CAD build for the part. Positions are in the model's coordinates, mm. A direction names the side the tool comes from. Give positions to 0.01 mm unless a question says otherwise; leave off trailing zeros. Write each loop counter-clockwise with the first axis right and the second up, starting at its lowest first coordinate (ties: lowest second). Pieces come first, ordered by that corner, then holes. Notation, with made-up numbers: (30.5, 18.5) - (77.5, 18.5) arc R36 cw to (77.5, 56.5) - close; hole circle Ø5 at (43, 64.5). An arc over 180 degrees is marked (long way). Put each result on its own line as item: value. Start each with the question number.
1. Wall check: line 1 (Y direction, x = 0, z = 0.6); line 2 (X direction, y = 12.5, z = 1.7); line 3 (Y direction, x = -21.5, z = 2.8). Give the ranges that are in metal, low to high.
2. Drop flat-ended pins along their axis: pin 1 (1 mm diameter, centred on y = 1.5, z = 0.5, fed in from -X); pin 2 (6.5 mm diameter, centred on x = -20.62, y = 11.91, fed in from -Z); pin 3 (1 mm diameter, centred on x = -0.5, z = 2, fed in from +Y); pin 4 (1 mm diameter, centred on x = -1.5, z = 1.5, fed in from -Y). Give the stop position or say it passes through.
3. Tool access for faces 4 (the flat face through (5.474, 3.219, 1.565)), 5 (the flat face through (0, 7, 0)): list every direction of +Z, -Z, +X, -X, +Y, -Y with a clear straight run to the whole face (end or side of a thin tool).
4. Mould opens along X. For faces 1 (the cylindrical face through (-30.133, 1.326, 1.565)), 2 (the flat face through (0, 7, 3.175)), 3 (the flat face through (5.525, -3.131, 1.565)) say: +X half, -X half, draft (parallel to the pull), parting line (faces both ways), or undercut.
5. Cut at D-D on y = 12.5. List the corners of the cut face in (x, z) (3 decimals).
6. Cut at B-B on y = 4.5. List the corners of the cut face in (x, z) (3 decimals).
7. Cut at A-A on x = 0. Give the number of separate pieces and of enclosed holes in the cut face, and give its area (3 significant figures).
from build123d import *

# Parameters (mm, degrees)
F0_R            = 30.1625
F1_DEPTH        = 3.175
F2_R            = 2.4892
F3_DEPTH        = 3.176
F3_COPIES_COUNT = 6
F4_R            = 2.3622
F5_DEPTH        = 3.176


# Not quite as in the source:
# - a pattern or mirror of a feature is missing from the dataset's text; its kind, count and spacing are read off the source's solid


with BuildPart() as f1:
    # F0 (on Top) → F1 (new body)
    with BuildSketch(Plane.XY):
        Circle(F0_R)
        Polygon((7.3323484187, 0), (3.6661742094, -6.35), (-3.6661742094, -6.35), (-7.3323484187, 0), (-3.6661742094, 6.35), (3.6661742094, 6.35), align=None, mode=Mode.SUBTRACT)
    extrude(amount=F1_DEPTH)

    # F2 (on face) → F3 (cut, through all)
    with BuildSketch(Plane.XY.offset(3.175)):
        with Locations((0, 23.8125)):
            Circle(F2_R)
    f3 = extrude(amount=-F3_DEPTH, mode=Mode.SUBTRACT)

    # F3_copies: F3 ×6 about axis
    f3_copies_axis = Axis((0, 0, 0), (0, 0, 1))
    for i in range(1, F3_COPIES_COUNT):
        add(f3.rotate(f3_copies_axis, i * 360 / F3_COPIES_COUNT), mode=Mode.SUBTRACT)

    # F4 (on face) → F5 (cut, through all)
    with BuildSketch(Plane.XY.offset(3.175)):
        with Locations((0, 40.2743678674)):
            Circle(F4_R)
        with Locations((38.3032, 12.4454641087)):
            Circle(F4_R)
        with Locations((23.6726794779, -32.5826480425)):
            Circle(F4_R)
        with Locations((-23.6726794779, -32.5826480425)):
            Circle(F4_R)
        with Locations((-38.3032, 12.4454641087)):
            Circle(F4_R)
    extrude(amount=-F5_DEPTH, mode=Mode.SUBTRACT)


solid = f1.part
Report:
1. line 1: y = -30.16 to -26.3, -21.32 to -6.35, 6.35 to 21.32, 26.3 to 30.16
1. line 2: x = -27.45 to -23.04, -18.2 to 18.2, 23.04 to 27.45
1. line 3: y = -21.15 to -14.24, -9.58 to 9.58, 14.24 to 21.15
2. pin 1: stops at x = -30.15
2. pin 2: stops at z = 0
2. pin 3: stops at y = 30.16
2. pin 4: stops at y = -30.15
3. face 4: +Z, -Z
3. face 5: -Z, +X, -X, +Y, -Y
4. face 1: parting line
4. face 2: draft
4. face 3: undercut
5. outline: (-27.45, 0) - (-23.04, 0) - (-23.04, 3.175) - (-27.45, 3.175) - close; (-18.205, 0) - (18.205, 0) - (18.205, 3.175) - (-18.205, 3.175) - close; (23.04, 0) - (27.45, 0) - (27.45, 3.175) - (23.04, 3.175) - close
6. outline: (-29.825, 0) - (-4.734, 0) - (-4.734, 3.175) - (-29.825, 3.175) - close; (4.734, 0) - (29.825, 0) - (29.825, 3.175) - (4.734, 3.175) - close
7. separate pieces: 4
7. enclosed holes: 0
7. area: 120 mm²
